```python
from build123d import *

# Parameters (mm, degrees)
SALIENTE_EXTRUIR1_DEPTH = 12
CROQUIS4_R              = 2.5
CORTAR_EXTRUIR1_DEPTH   = 1
CROQUIS5_R              = 1.5
CORTAR_EXTRUIR2_DEPTH   = 1
CROQUIS6_W              = 13
CROQUIS6_H              = 1
CORTAR_EXTRUIR3_DEPTH   = 12


with BuildPart() as part:
    # Croquis1 → Saliente-Extruir1 (new body)
    with BuildSketch(Plane(origin=(0, 0, 0), x_dir=(1, 0, 0), z_dir=(0, 1, 0))):
        Polygon((-65.844332906, 24.038216561), (83.155667094, 24.038216561), (83.155667094, 26.038216561), (-65.844332906, 26.038216561), (-68.344332906, 26.038216561), (-68.344332906, 24.038216561), align=None)
    extrude(amount=SALIENTE_EXTRUIR1_DEPTH)

    # Croquis4 → Cortar-Extruir1 (cut)
    with BuildSketch(Plane.XY.offset(-24.038216561)):
        with Locations((79.155667094, 6)):
            Circle(CROQUIS4_R)
    extrude(amount=-CORTAR_EXTRUIR1_DEPTH, mode=Mode.SUBTRACT)

    # Croquis5 → Cortar-Extruir2 (cut)
    with BuildSketch(Plane.XY.offset(-25.038216561)):
        with Locations((79.155667094, 6)):
            Circle(CROQUIS5_R)
    extrude(amount=-CORTAR_EXTRUIR2_DEPTH, mode=Mode.SUBTRACT)

    # Croquis6 → Cortar-Extruir3 (cut)
    with BuildSketch(Plane(origin=(0, 12, 0), x_dir=(1, 0, 0), z_dir=(0, 1, 0))):
        with Locations((76.655667094, 25.538216561)):
            Rectangle(CROQUIS6_W, CROQUIS6_H)
    extrude(amount=-CORTAR_EXTRUIR3_DEPTH, mode=Mode.SUBTRACT)


solid = part.part
```
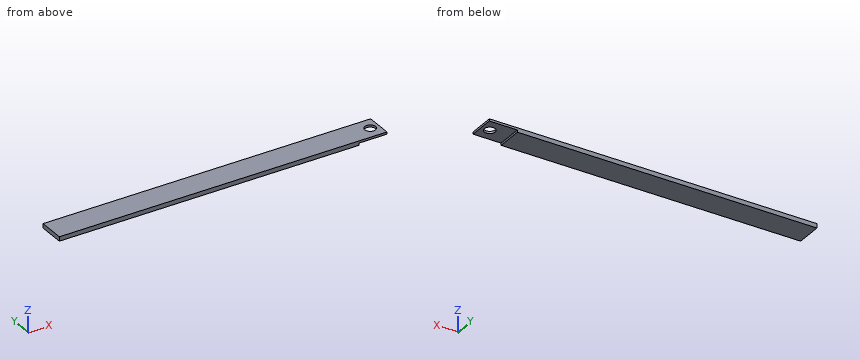
Work out the finished part from the listing and answer in its coordinate system (mm). Give positions to 0.01 mm unless a question says otherwise; leave off trailing zeros. Write each loop counter-clockwise with the first axis right and the second up, starting at its lowest first coordinate (ties: lowest second). Pieces come first, ordered by that corner, then holes. Notation, with made-up numbers: (65.25, -30.5) - (81.25, -30.5) arc R17 cw to (81.25, -4.5) - close; hole circle Ø2 at (-35.5, 27). An arc over 180 degrees is marked (long way). Use one line per item in the form item = value.
1. This flat-tipped pin is pushed along its axis until it touches: pin 1 Ø6 at (x, y) = (79.16, 6) entering from +Z. Where does it stop, or does it pass through?
Filled in:
pin_1 = -24.04
2. A cutting plane is placed at A-A (y = 6). Write down the section's boundary in (x, z).
Filled in:
outline = (-68.34, -26.04) - (70.16, -26.04) - (70.16, -25.04) - (76.66, -25.04) - (76.66, -24.04) - (-68.34, -24.04) - close; (81.66, -25.04) - (83.16, -25.04) - (83.16, -24.04) - (81.66, -24.04) - close
3. Consider L1, parallel to X at y = 1.25, z = -25.65; L2, parallel to X at y = 7.5, z = -24.5. Determine where each line is inside the solid, lowest interval first.
Filled in:
L1 = -68.34 to 70.16
L2 = -68.34 to 77.16, 81.16 to 83.16
4. A cutting plane is placed at B-B (z = -25.5). Write down the section's boundary in (x, y), and give its area (3 significant figures).
Filled in:
outline = (-68.34, 0) - (70.16, 0) - (70.16, 12) - (-68.34, 12) - close
area = 1,660 mm^2
